from build123d import *

# Parameters (mm, degrees)
SKETCH_R     = 5.15
SKETCH_R_2   = 3
PAD_DEPTH    = 20
SKETCH001_R  = 3
PAD001_DEPTH = 0.8
FILLET_R     = 0.4
FILLET001_R  = 0.4
FILLET002_R  = 0.4
CHAMFER_SIZE = 1


with BuildPart() as part:
    # Sketch → Pad (new body)
    with BuildSketch(Plane.XY):
        Circle(SKETCH_R)
        Circle(SKETCH_R_2, mode=Mode.SUBTRACT)
    extrude(amount=PAD_DEPTH)

    # Sketch001 (on Face3 of Pad) → Pad001 (join)
    with BuildSketch(Plane(origin=(0, 0, 0), x_dir=(1, 0, 0), z_dir=(0, 0, -1))):
        with BuildLine():
            ThreePointArc((2.478578, 6.809837), (3.535332, 4.213244), (6.27598, 3.623438))
            ThreePointArc((6.27598, 3.623438), (5.416443, 0.955065), (7.136781, -1.258407))
            ThreePointArc((7.136781, -1.258407), (4.76314, -2.75), (4.658203, -5.55143))
            ThreePointArc((4.658203, -5.55143), (1.881111, -5.168309), (0, -7.246877))
            ThreePointArc((0, -7.246877), (-1.881111, -5.168309), (-4.658203, -5.55143))
            ThreePointArc((-4.658203, -5.55143), (-4.76314, -2.75), (-7.136781, -1.258407))
            ThreePointArc((-7.136781, -1.258407), (-5.416443, 0.955065), (-6.27598, 3.623438))
            ThreePointArc((-6.27598, 3.623438), (-3.535332, 4.213244), (-2.478578, 6.809837))
            ThreePointArc((-2.478578, 6.809837), (0, 5.5), (2.478578, 6.809837))
        make_face()
        Circle(SKETCH001_R, mode=Mode.SUBTRACT)
    extrude(amount=PAD001_DEPTH)

    # Fillet
    fillet_edges = [part.edges().sort_by_distance(p)[0] for p in [
        (-2.478578, -6.809837, -0.4),
    ]]
    fillet(fillet_edges, radius=FILLET_R)

    # Fillet001
    fillet001_edges = [part.edges().sort_by_distance(p)[0] for p in [
        (2.478578, -6.809837, -0.4),
        (6.27598, -3.623438, -0.4),
        (-6.27598, -3.623438, -0.4),
        (-7.136781, 1.258407, -0.4),
        (-4.658203, 5.55143, -0.4),
        (0, 7.246877, -0.4),
    ]]
    fillet(fillet001_edges, radius=FILLET001_R)

    # Fillet002
    fillet002_edges = [part.edges().sort_by_distance(p)[0] for p in [
        (4.658203, 5.55143, -0.4),
        (7.136781, 1.258407, -0.4),
    ]]
    fillet(fillet002_edges, radius=FILLET002_R)

    # Chamfer
    chamfer_edges = [part.edges().sort_by_distance(p)[0] for p in [
        (-5.15, 0, 20),
    ]]
    chamfer(chamfer_edges, length=CHAMFER_SIZE)


solid = part.part
Design review of the part built by this model. Coordinates are the model's own, in mm. A direction names the side the tool comes from. Give positions to 0.01 mm unless a question says otherwise; leave off trailing zeros. Order: outer loops, then holes, each group sorted by start corner. A loop starts at its lowest first (then second) coordinate and runs counter-clockwise, first axis right, second up.
1. For pin 1 Ø4 at (y, z) = (5, 12) entering from +X; pin 2 Ø1 at (y, z) = (4.5, 13.5) entering from +X; pin 3 Ø5 at (y, z) = (2.5, 16.5) entering from -X, all flat-tipped, find the tip position at first contact; note any pin that passes through.
Solution:
pin 1: stops at x = 4.19
pin 2: stops at x = 3.24
pin 3: stops at x = -5.15
2. Add section B-B, the plane z = 16.25. State the section outline as (x, y) points.
Solution:
outline: circle Ø10.3 at (0, 0); hole circle Ø6 at (0, 0)
3. To check wall thickness, follow L1, parallel to Y at x = 0, z = 8.5; L2, parallel to Y at x = 2.75, z = 5.5; L3, parallel to X at y = 2, z = 1.25. State the ranges of each line that lie inside material, in increasing order.
Solution:
L1: y = -5.15 to -3, 3 to 5.15
L2: y = -4.35 to -1.2, 1.2 to 4.35
L3: x = -4.75 to -2.24, 2.24 to 4.75
4. Mouldability with a two-part tool opening along Y and no side actions: class faces 3 (the cylindrical face through (-3.557, -4.195, -0.394)), 4 (the cylindrical face through (4.777, 2.725, -0.394)), 5 (the cylindrical face through (-1.85, 5.18, -0.39)) as +Y half, -Y half, draft (parallel to the pull), parting line (faces both ways), or undercut.
Solution:
face 3: -Y half
face 4: undercut
face 5: +Y half
5. Tool access review of faces 1 (the cylindrical face through (1.91, 5.16, -0.39)), 2 (the flat face through (2, -5, 0)): name each direction out of +Z, -Z, +X, -X, +Y, -Y from which nothing blocks a thin tool from reaching the whole face with its end or side.
Solution:
face 1: +Z, -Z, +Y
face 2: +Z
6. Add section A-A, the plane y = 0. State the section outline as (x, z) points.
Solution:
outline: (-5.76, -0.8) - (-3, -0.8) - (-3, 20) - (-4.15, 20) - (-5.15, 19) - (-5.15, 0) - (-5.76, 0) - close; (3, -0.8) - (5.76, -0.8) - (5.76, 0) - (5.15, 0) - (5.15, 19) - (4.15, 20) - (3, 20) - close
